Could you check a few things on this model? Use its own coordinates, in mm. Face numbers are marked on the shaded views. A direction names the side the tool comes from. Round coordinates to 2 decimals unless told otherwise and drop trailing zeros. Write each loop counter-clockwise with the first axis right and the second up, starting at its lowest first coordinate (ties: lowest second). Pieces come first, ordered by that corner, then holes. Notation, with made-up numbers: (75, 9) -> (81, 9) arc R18 cw to (81, 30) -> close; hole circle Ø10 at (6, 62.25). An arc over 180 degrees is marked (long way). Return JSON: item names as keys, results as strings.
from build123d import *

# Parameters (mm, degrees)
SKETCH1_R                = 12
BOSS_EXTRUDE1_DEPTH      = 10.25
SKETCH4_W                = 19.75
SKETCH4_H                = 16.5
BOSS_EXTRUDE4_DEPTH      = 1.6
SKETCH5_OUTSIDE_W        = 33.728
SKETCH5_OUTSIDE_H        = 38.228
SKETCH5_OUTSIDE_R        = 16.5
CUT_EXTRUDE1_DEPTH       = 1.6
FILLET2_R                = 2
SKETCH6_W                = 3
SKETCH6_H                = 12.32415633
BOSS_EXTRUDE6_DEPTH      = 0.5
FILLET3_R                = 1
CIRPATTERN1_COUNT        = 2
CIRPATTERN1_ANGLE        = 25
FILLET3_OF_CIRPATTERN1_R = 1
CIRPATTERN2_COUNT        = 2
CIRPATTERN2_ANGLE        = 25
FILLET3_OF_CIRPATTERN2_R = 1
SKETCH2_R                = 4.625
BOSS_EXTRUDE2_DEPTH      = 9.6
SKETCH3_R                = 9.2
BOSS_EXTRUDE3_DEPTH      = 18
BOSS_EXTRUDE7_DEPTH      = 4


with BuildPart() as part:
    # Sketch1 → Boss-Extrude1 (new body)
    with BuildSketch(Plane(origin=(0, 0, 0), x_dir=(1, 0, 0), z_dir=(0, 1, 0))):
        Circle(SKETCH1_R)
    extrude(amount=BOSS_EXTRUDE1_DEPTH)

    # Sketch4 → Boss-Extrude4 (add)
    with BuildSketch(Plane(origin=(0, 10.25, 0), x_dir=(1, 0, 0), z_dir=(0, 1, 0))):
        with Locations((0, -8.25)):
            Rectangle(SKETCH4_W, SKETCH4_H)
    extrude(amount=-BOSS_EXTRUDE4_DEPTH)

    # Sketch5 outside → Cut-Extrude1 (cut)
    with BuildSketch(Plane(origin=(0, 10.25, 0), x_dir=(1, 0, 0), z_dir=(0, 1, 0))):
        with Locations((0, -2.25)):
            Rectangle(SKETCH5_OUTSIDE_W, SKETCH5_OUTSIDE_H)
        Circle(SKETCH5_OUTSIDE_R, mode=Mode.SUBTRACT)
    extrude(amount=-CUT_EXTRUDE1_DEPTH, mode=Mode.SUBTRACT)

    # Fillet2
    fillet2_edges = [part.edges().sort_by_distance(p)[0] for p in [
        (-9.875, 9.45, 13.218713061),
        (9.875, 9.45, 13.218713061),
    ]]
    fillet(fillet2_edges, radius=FILLET2_R)

    # Sketch6 → Boss-Extrude6 (add)
    with BuildSketch(Plane.XZ.offset(-8.65)):
        with Locations((0, 18.837921835)):
            Rectangle(SKETCH6_W, SKETCH6_H)
    boss_extrude6 = extrude(amount=BOSS_EXTRUDE6_DEPTH)

    # Fillet3
    fillet3_edges = [part.edges().sort_by_distance(p)[0] for p in [
        (-1.5, 8.4, 25),
        (1.5, 8.4, 25),
    ]]
    fillet(fillet3_edges, radius=FILLET3_R)

    # CirPattern1: Boss-Extrude6 ×2 about axis
    cirpattern1_axis = Axis((0, 0, 0), (0, 1, 0))
    for i in range(1, CIRPATTERN1_COUNT):
        add(boss_extrude6.rotate(cirpattern1_axis, i * CIRPATTERN1_ANGLE / (CIRPATTERN1_COUNT - 1)))

    # Fillet3 of CirPattern1
    fillet3_of_cirpattern1_edges = [part.edges().sort_by_distance(p)[0] for p in [
        (9.205994863, 8.4, 23.291622069),
        (11.924918224, 8.4, 22.023767283),
    ]]
    fillet(fillet3_of_cirpattern1_edges, radius=FILLET3_OF_CIRPATTERN1_R)

    # CirPattern2: Boss-Extrude6 ×2 about axis
    cirpattern2_axis = Axis((0, 0, 0), (0, -1, 0))
    for i in range(1, CIRPATTERN2_COUNT):
        add(boss_extrude6.rotate(cirpattern2_axis, i * CIRPATTERN2_ANGLE / (CIRPATTERN2_COUNT - 1)))

    # Fillet3 of CirPattern2
    fillet3_of_cirpattern2_edges = [part.edges().sort_by_distance(p)[0] for p in [
        (-11.924918224, 8.4, 22.023767283),
        (-9.205994863, 8.4, 23.291622069),
    ]]
    fillet(fillet3_of_cirpattern2_edges, radius=FILLET3_OF_CIRPATTERN2_R)

    # Sketch2 → Boss-Extrude2 (add)
    with BuildSketch(Plane(origin=(0, 10.25, 0), x_dir=(1, 0, 0), z_dir=(0, 1, 0))):
        Circle(SKETCH2_R)
    extrude(amount=BOSS_EXTRUDE2_DEPTH)

    # Sketch3 → Boss-Extrude3 (add)
    with BuildSketch(Plane(origin=(0, 19.85, 0), x_dir=(1, 0, 0), z_dir=(0, 1, 0))):
        Circle(SKETCH3_R)
    extrude(amount=BOSS_EXTRUDE3_DEPTH)

    # Sketch7 → Boss-Extrude7 (add)
    with BuildSketch(Plane(origin=(0, 10.25, 0), x_dir=(1, 0, 0), z_dir=(0, 1, 0))):
        with BuildLine():
            Line((-11.9058809, 1.5), (-10.665684973, 1.34375))
            ThreePointArc((-10.665684973, 1.34375), (-10.75, 0), (-10.665684973, -1.34375))
            Line((-10.665684973, -1.34375), (-11.9058809, -1.5))
            ThreePointArc((-11.9058809, -1.5), (-12, 0), (-11.9058809, 1.5))
        make_face()
    extrude(amount=BOSS_EXTRUDE7_DEPTH)


solid = part.part
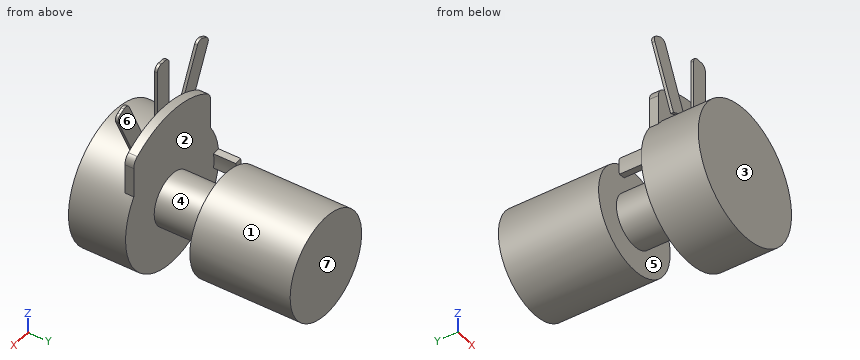
1) I want a section at C-C, the plane z = 0. Please give me the cut outline in (x, y) (3 decimals).
Return value:
{"outline": "(-12, 0) -> (12, 0) -> (12, 10.25) -> (4.625, 10.25) -> (4.625, 19.85) -> (9.2, 19.85) -> (9.2, 37.85) -> (-9.2, 37.85) -> (-9.2, 19.85) -> (-4.625, 19.85) -> (-4.625, 10.25) -> (-10.75, 10.25) -> (-10.75, 14.25) -> (-12, 14.25) -> close"}
2) I want a section at A-A, the plane x = 0. Please give me the cut outline in (y, z) (3 decimals).
Return value:
{"outline": "(0, -12) -> (10.25, -12) -> (10.25, -4.625) -> (19.85, -4.625) -> (19.85, -9.2) -> (37.85, -9.2) -> (37.85, 9.2) -> (19.85, 9.2) -> (19.85, 4.625) -> (10.25, 4.625) -> (10.25, 16.5) -> (8.65, 16.5) -> (8.65, 25) -> (8.15, 25) -> (8.15, 12.676) -> (8.65, 12.676) -> (8.65, 12) -> (0, 12) -> close"}
3) If I drill on probe 1 along Z at (x, y) = (0, 8.5); probe 2 along Y at (x, z) = (-4.5, -5); probe 3 along Y at (x, z) = (-4.5, -11), over which ranges is the centre line in solid material (lowest first)? Write a range as [from, to].
Return value:
{"probe 1": "[-12, 12], [12.68, 25]", "probe 2": "[0, 10.25], [19.85, 37.85]", "probe 3": "[0, 10.25]"}
4) Will these pins go through, and if not, where does the flat tip stop? pin 1 Ø2 at (x, y) = (5.5, 4.5) entering from -Z; pin 2 Ø1.5 at (x, y) = (1.5, 9.5) entering from -Z; pin 3 Ø6 at (x, z) = (6, 20) entering from -Y; pin 4 Ø8 at (y, z) = (31.5, 14.5) entering from +X.
Return value:
{"pin 1": "z = -11.12", "pin 2": "z = -11.98", "pin 3": "y = 8.15", "pin 4": "through"}
5) I want a section at D-D, the plane z = 8.5. Please give me the cut outline in (x, y) (3 decimals).
Return value:
{"outline": "(-9.875, 8.65) -> (-8.471, 8.65) -> (-8.471, 0) -> (8.471, 0) -> (8.471, 8.65) -> (9.875, 8.65) -> (9.875, 10.25) -> (-9.875, 10.25) -> close; (-3.52, 19.85) -> (3.52, 19.85) -> (3.52, 37.85) -> (-3.52, 37.85) -> close"}
6) Thinking about a two-plate mould opening in Y: for the marked faces 1, 2, 3 and 4, which applies, pulls with the +Y half, pulls with the -Y half, needs draft (parallel to the pull), parting line crosses it, or undercut?
Return value:
{"face 1": "needs draft", "face 2": "undercut", "face 3": "pulls with the -Y half", "face 4": "undercut"}
7) I want a section at B-B, the plane z = 19.5. Please give me the cut outline in (x, y), and give its area (3 significant figures).
Return value:
{"outline": "(-10.75, 8.15) -> (-7.44, 8.15) -> (-7.44, 8.65) -> (-10.75, 8.65) -> close; (-1.5, 8.15) -> (1.5, 8.15) -> (1.5, 8.65) -> (-1.5, 8.65) -> close; (7.44, 8.15) -> (10.75, 8.15) -> (10.75, 8.65) -> (7.44, 8.65) -> close", "area": "4.81 mm²"}
8) For the marked faces 5, 6 and 7, which set-ups out of +Z, -Z, +X, -X, +Y, -Y let a thin tool reach every point of the face, with its end or its side?
Return value:
{"face 5": "none", "face 6": "+Z, +X, +Y", "face 7": "+Z, -Z, +X, -X, +Y"}
